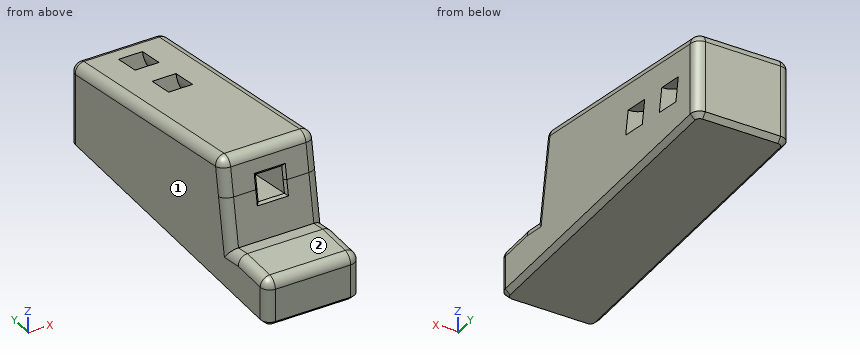
from build123d import *

# Parameters (mm, degrees)
SKETCH003_R             = 6.25
SKETCH003_R_2           = 3.75
PAD002_DEPTH            = 3
BODY002_PLACEMENT_ANGLE = 350
PAD_DEPTH               = 9.88
SKETCH001_W             = 2.75
SKETCH001_H             = 2.75
POCKET_DEPTH            = 20
FILLET_R                = 1
CHAMFER_SIZE            = 0.5
CHAMFER001_SIZE         = 0.25


with BuildPart() as obj1:
    # Sketch003 → Pad002 (new body)
    with BuildSketch(Plane.XZ):
        Circle(SKETCH003_R)
        Circle(SKETCH003_R_2, mode=Mode.SUBTRACT)
    extrude(amount=-PAD002_DEPTH)


with BuildPart() as obj1_1:
    # Body002 placement: moved
    add(obj1.part.moved(Location((-24.4, 17, 6.25))).rotate(Axis((-24.4, 17, 6.25), (1, 0, 0)), BODY002_PLACEMENT_ANGLE))


with BuildPart() as obj2:
    # Body003 base: copy of obj1
    add(obj1_1.part)


with BuildPart() as obj2_1:
    # Body003 placement: moved
    add(obj2.part.moved(Location((0, 6, -1))))


with BuildPart() as foot_w_cuts:
    # Sketch → Pad (new body)
    with BuildSketch(Plane.YZ):
        Polygon((1.57769, 8.947526), (0.883098, 5.008295), (0, 0), (-1.575692, 0.277837), (-6.575692, 0.277837), (-6.575692, -4.722163), (28.424308, -4.722163), (28.424308, 4.213743), align=None)
    extrude(amount=PAD_DEPTH)

    # Sketch001 (on Face9 of Pad) → Pocket (cut)
    with BuildSketch(Plane(origin=(0, 0, 0), x_dir=(0, -0.173648, -0.984808), z_dir=(0, -0.984808, 0.173648))):
        with Locations((-5.087502, 4.946713)):
            Rectangle(SKETCH001_W, SKETCH001_H)
    extrude(amount=-POCKET_DEPTH, mode=Mode.SUBTRACT)

    # Fillet
    fillet_edges = [foot_w_cuts.edges().sort_by_distance(p)[0] for p in [
        (9.88, -4.075692, 0.277837),
        (4.94, -6.575692, 0.277837),
        (0, -4.075692, 0.277837),
        (4.94, 1.57769, 8.947526),
        (0, 15.000999, 6.580635),
        (9.88, 15.000999, 6.580635),
        (9.88, 0.788845, 4.473763),
        (0, 0.788845, 4.473763),
        (4.94, 28.424308, 4.213743),
        (9.88, 28.424308, -0.25421),
        (9.88, -0.787846, 0.138919),
        (0, -0.787846, 0.138919),
        (9.88, -6.575692, -2.222163),
        (0, -6.575692, -2.222163),
        (0, 28.424308, -0.25421),
    ]]
    fillet(fillet_edges, radius=FILLET_R)

    # Chamfer
    chamfer_edges = [foot_w_cuts.edges().sort_by_distance(p)[0] for p in [
        (0, 10.924308, -4.722163),
    ]]
    chamfer(chamfer_edges, length=CHAMFER_SIZE)

    # Chamfer001
    chamfer001_edges = [foot_w_cuts.edges().sort_by_distance(p)[0] for p in [
        (3.571713, 0.883435, 5.010211),
        (4.946713, 1.122202, 6.364322),
        (6.321713, 0.883435, 5.010211),
        (4.946713, 0.644669, 3.656101),
    ]]
    chamfer(chamfer001_edges, length=CHAMFER001_SIZE)


with BuildPart() as foot_w_cuts_1:
    # Body placement: moved
    add(foot_w_cuts.part.moved(Location((-34.3, 0, 0))))

    # Cut: cut obj1
    add(obj1_1.part, mode=Mode.SUBTRACT)

    # Cut001: cut obj2
    add(obj2_1.part, mode=Mode.SUBTRACT)


solid = foot_w_cuts_1.part
Here's how the part is built. I have some questions about the finished solid (model axes, mm). Face numbers are marked on the shaded views. A direction names the side the tool comes from. Give positions to 0.01 mm unless a question says otherwise; leave off trailing zeros. Order: outer loops, then holes, each group sorted by start corner. A loop starts at its lowest first (then second) coordinate and runs counter-clockwise, first axis right, second up. Notation, with made-up numbers: M -16,78.5 L 29,78.5 A22 ccw 29,100.5 Z; hole C -6,49 d5. An arc over 180 degrees is marked long. Answer as a JSON object with one key per item and string values. Group by question number.
1) On a 3-axis mill with a long thin cutter (end or side, diameter ignored), from which of +Z, -Z, +X, -X, +Y, -Y can I reach the whole of each face in a straight line? I mean the marked faces 1 and 2. Say none if no direction works.
2) Suppose I cut it at B-B, the plane y = -4. Write out the boundary of the cut face in (x, z).
3) Please list where these lines run through material, in increasing order: L1, parallel to X at y = 5, z = 3.5; L2, parallel to Z at x = -30.5, y = -3.5; L3, parallel to Z at x = -29.5, y = 5. Write a range as [from, to].
4) I'm going to push flat-ended pins straight in: pin 1 Ø1.2 at (x, y) = (-27.5, -3) entering from +Z; pin 2 Ø5 at (x, y) = (-26.5, 21) entering from +Z. Where does each tip first touch, or does it pass through?
5) Suppose I cut it at C-C, the plane x = -27. Write out the boundary of the cut face in (y, z).
6) Suppose I cut it at A-A, the plane x = -31.5. Write out the boundary of the cut face in (y, z), plus the area to 3 significant figures.
Results found:
{
 "1": {"face 1": "+Z, -Z, -X, +Y, -Y", "face 2": "+Z, +X, -X, -Y"},
 "2": {"outline": "M -34.3,-4.22 L -33.8,-4.72 L -24.92,-4.72 L -24.42,-4.22 L -24.42,-0.72 A1 ccw -25.42,0.28 L -33.3,0.28 A1 ccw -34.3,-0.72 Z"},
 "3": {"L1": "[-34.3, -30.73], [-27.98, -24.42]", "L2": "[-4.72, 0.28]", "L3": "[-4.72, 2.89], [5.68, 8.34]"},
 "4": {"pin 1": "z = 0.28", "pin 2": "z = 5.96"},
 "5": {"outline": "M -6.58,-4.22 L -6.08,-4.72 L 27.92,-4.72 L 28.42,-4.22 L 28.42,3.37 A1 ccw 27.6,4.36 L 2.56,8.77 A1 ccw 1.4,7.96 L 0.88,5.01 L 0,0 L -1.58,0.28 L -5.58,0.28 A1 ccw -6.58,-0.72 Z; hole M 16.01,0.65 L 18.97,0.13 L 19.49,3.07 L 16.53,3.59 Z; hole M 22.01,-0.35 L 24.97,-0.87 L 25.49,2.07 L 22.53,2.59 Z"},
 "6": {"outline": "M -6.58,-4.22 L -6.08,-4.72 L 27.92,-4.72 L 28.42,-4.22 L 28.42,3.37 A1 ccw 27.6,4.36 L 2.56,8.77 A1 ccw 1.4,7.96 L 0.88,5.01 L 0,0 L -1.58,0.28 L -5.58,0.28 A1 ccw -6.58,-0.72 Z", "area": "350 mm²"}
}
